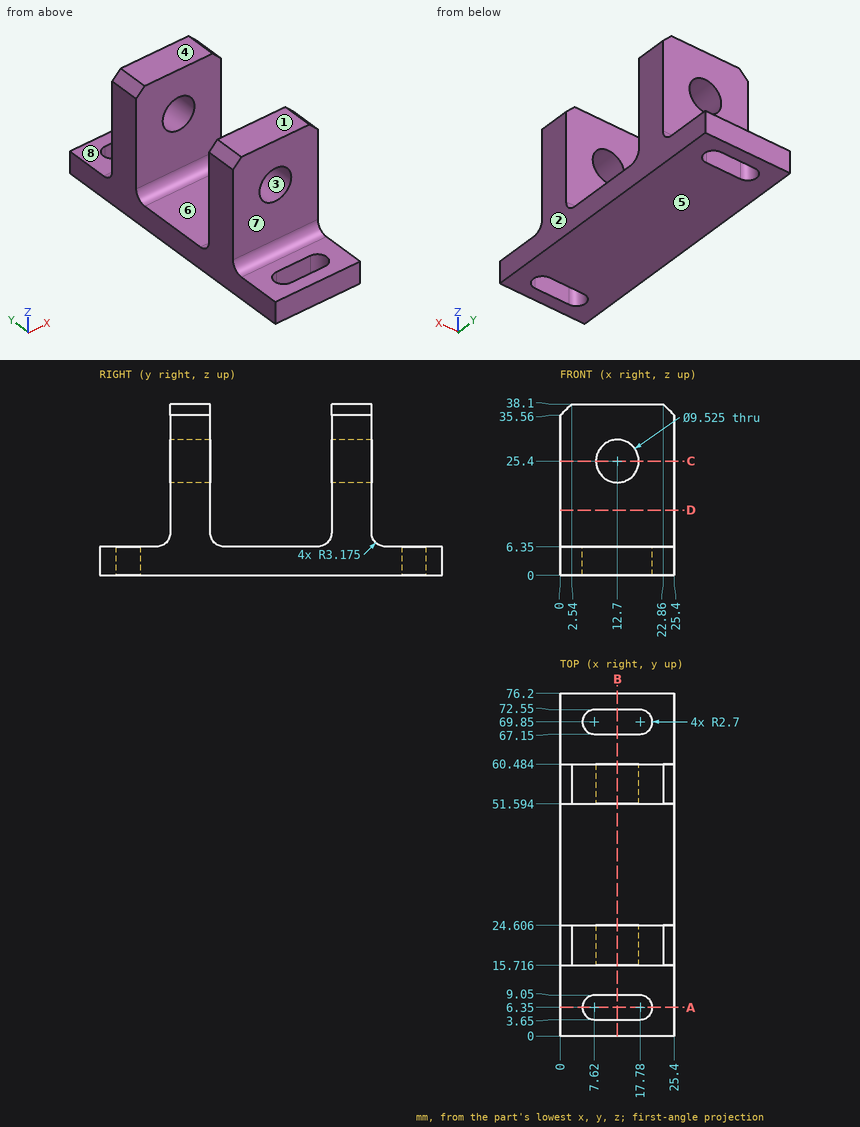
Verification items for this drawing (mm, ordinates from the low corner). A direction names the side the tool comes from. Coordinates: 2 decimals unless noted, no trailing zeros. Order: outer loops, then holes, each group sorted by start corner. A loop starts at its lowest first (then second) coordinate and runs counter-clockwise, first axis right, second up.
Q1. Sectioned sample at A-A on y = 6.35. Record the cut outline in (x, z).
Reply:
outline: (0, 0) - (4.92, 0) - (4.92, 6.35) - (0, 6.35) - close; (20.48, 0) - (25.4, 0) - (25.4, 6.35) - (20.48, 6.35) - close
Q2. Sectioned sample at C-C on z = 25.4. Record the cut outline in (x, y).
Reply:
outline: (0, 15.72) - (7.94, 15.72) - (7.94, 24.61) - (0, 24.61) - close; (0, 51.59) - (7.94, 51.59) - (7.94, 60.48) - (0, 60.48) - close; (17.46, 15.72) - (25.4, 15.72) - (25.4, 24.61) - (17.46, 24.61) - close; (17.46, 51.59) - (25.4, 51.59) - (25.4, 60.48) - (17.46, 60.48) - close
Q3. Sectioned sample at B-B on x = 12.7. Give the number of separate pieces and of enclosed holes in the cut face, and give its area (3 significant figures).
Reply:
separate pieces: 5
enclosed holes: 0
area: 819 mm2
Q4. Tool access check on the marked faces 4, 5, 6, 7 and 8. Record the directions out of +Z, -Z, +X, -X, +Y, -Y that give a thin tool (end or side, any length) a straight path to the whole face; none if there is none.
Reply:
face 4: +Z, +X, -X, +Y, -Y
face 5: -Z, +X, -X, +Y, -Y
face 6: +Z, +X, -X
face 7: +Z, +X, -X, -Y
face 8: +Z, +X, -X, +Y
Q5. Depth check by flat-ended pin: pin 1 Ø7.5 at (x, z) = (9.5, 25.5) entering from +Y; pin 2 Ø6.5 at (x, y) = (6.5, 67) entering from +Z; pin 3 Ø12.5 at (x, z) = (12.7, 25.4) entering from -Y; pin 4 Ø10 at (y, z) = (66.5, 18.5) entering from +X. Enter the tip coordinate at first touch or a pass-through.
Reply:
pin 1: stops at y = 60.48
pin 2: stops at z = 6.35
pin 3: stops at y = 15.72
pin 4: passes through
Q6. Thickness scan on probe 1 along Y at (x, z) = (18, 4.5); probe 2 along Y at (x, z) = (17.5, 33); probe 3 along Z at (x, y) = (12.7, 56). Record the ranges inside material, lowest first.
Reply:
probe 1: y = 0 to 3.66, 9.04 to 67.16, 72.54 to 76.2
probe 2: y = 15.72 to 24.61, 51.59 to 60.48
probe 3: z = 0 to 20.64, 30.16 to 38.1
Q7. Draft check along Z on the marked faces 1, 2 and 3. Enter one of: released by +Z, released by -Z, zero draft, split by the parting line, or undercut.
Reply:
face 1: released by +Z
face 2: zero draft
face 3: undercut
Q8. Sectioned sample at D-D on z = 14.5. Record the cut outline in (x, y), and give its area (3 significant figures).
Reply:
outline: (0, 15.72) - (25.4, 15.72) - (25.4, 24.61) - (0, 24.61) - close; (0, 51.59) - (25.4, 51.59) - (25.4, 60.48) - (0, 60.48) - close
area: 452 mm2
